from build123d import *

# Parameters (mm, degrees)
BOSS_EXTRUDE1_DEPTH     = 203.2
CUT_EXTRUDE3_DEPTH      = 17.51
CUT_EXTRUDE3_DEPTH_BACK = 4.175
SKETCH7_R               = 3.683
SKETCH7_R_2             = 1.63195
CUT_EXTRUDE4_DEPTH      = 20.685
SKETCH8_R               = 1.89865
CUT_EXTRUDE5_DEPTH      = 4.175
SKETCH9_R               = 1.89865
CUT_EXTRUDE6_DEPTH      = 4.175
SKETCH10_R              = 1.7526
CUT_EXTRUDE7_DEPTH      = 4.175
BOSS_EXTRUDE2_DEPTH     = 3.175
SKETCH12_R              = 2.54
CUT_EXTRUDE8_DEPTH      = 4.175
SKETCH13_R              = 1.89865
CUT_EXTRUDE9_DEPTH      = 4.175


with BuildPart() as part:
    # Sketch1 → Boss-Extrude1 (new body)
    with BuildSketch(Plane(origin=(0, 0, 0), x_dir=(1, 0, 0), z_dir=(0, 1, 0))):
        Polygon((0, 0), (-19.685, 0), (-19.685, 3.175), (-3.175, 3.175), (-3.175, 50.8), (0, 50.8), align=None)
    extrude(amount=BOSS_EXTRUDE1_DEPTH)

    # Sketch5 → Cut-Extrude3 (cut, two sides)
    with BuildSketch(Plane.ZY.offset(3.175)) as cut_extrude3_sk:
        Polygon((0, 163.322), (-50.8, 214.122), (-60.823247691, 214.122), (-60.823247691, 256.047203652), (33.196571846, 256.047203652), (33.196571846, 163.322), align=None)
    extrude(amount=CUT_EXTRUDE3_DEPTH, mode=Mode.SUBTRACT)
    extrude(cut_extrude3_sk.sketch, amount=-CUT_EXTRUDE3_DEPTH_BACK, mode=Mode.SUBTRACT)

    # Sketch7 → Cut-Extrude4 (cut, through all)
    with BuildSketch(Plane(origin=(0, 0, 0), x_dir=(0, 0, -1), z_dir=(1, 0, 0))):
        with Locations((25.4, 152.4)):
            Circle(SKETCH7_R)
        with Locations((25.4, 160.782)):
            Circle(SKETCH7_R_2)
        with Locations((25.4, 144.018)):
            Circle(SKETCH7_R_2)
    extrude(amount=-CUT_EXTRUDE4_DEPTH, mode=Mode.SUBTRACT)

    # Sketch8 → Cut-Extrude5 (cut, through all)
    with BuildSketch(Plane.ZY.offset(3.175)):
        with Locations((-30.48, 182.88)):
            Circle(SKETCH8_R)
        with Locations((-30.48, 8.89)):
            Circle(SKETCH8_R)
    extrude(amount=-CUT_EXTRUDE5_DEPTH, mode=Mode.SUBTRACT)

    # Sketch9 → Cut-Extrude6 (cut, through all)
    with BuildSketch(Plane.ZY.offset(3.175)):
        with Locations((-19.05, 40.577339992)):
            Circle(SKETCH9_R)
        with Locations((-19.05, 124.397339992)):
            Circle(SKETCH9_R)
    extrude(amount=-CUT_EXTRUDE6_DEPTH, mode=Mode.SUBTRACT)

    # Sketch10 → Cut-Extrude7 (cut, through all)
    with BuildSketch(Plane(origin=(0, 0, -3.175), x_dir=(-1, 0, 0), z_dir=(0, 0, -1))):
        with Locations((9.525, 11.43)):
            Circle(SKETCH10_R)
        with Locations((9.525, 150.603948776)):
            Circle(SKETCH10_R)
    extrude(amount=-CUT_EXTRUDE7_DEPTH, mode=Mode.SUBTRACT)

    # Sketch11 → Boss-Extrude2 (add)
    with BuildSketch(Plane(origin=(0, 0, 0), x_dir=(0, 0, -1), z_dir=(1, 0, 0))):
        Polygon((0, 228.6), (0, 163.322), (39.878, 203.2), (50.8, 203.2), (50.8, 228.6), align=None)
    extrude(amount=-BOSS_EXTRUDE2_DEPTH)

    # Sketch12 → Cut-Extrude8 (cut, through all)
    with BuildSketch(Plane.ZY.offset(3.175)):
        with Locations((-33.136196499, 25.4)):
            Circle(SKETCH12_R)
    extrude(amount=-CUT_EXTRUDE8_DEPTH, mode=Mode.SUBTRACT)

    # Sketch13 → Cut-Extrude9 (cut, through all)
    with BuildSketch(Plane.ZY.offset(3.175)):
        with Locations((-43.18, 12.7)):
            Circle(SKETCH13_R)
        with Locations((-43.18, 190.498941664)):
            Circle(SKETCH13_R)
    extrude(amount=-CUT_EXTRUDE9_DEPTH, mode=Mode.SUBTRACT)


solid = part.part
CAD build for the part. Positions are in the model's coordinates, mm. A direction names the side the tool comes from. Round coordinates to 2 decimals unless told otherwise and drop trailing zeros. Order: outer loops, then holes, each group sorted by start corner. A loop starts at its lowest first (then second) coordinate and runs counter-clockwise, first axis right, second up. Notation, with made-up numbers: (50, 7) -> (82, 7) arc R20 cw to (82, 38) -> close; hole circle Ø5 at (-26, 86). An arc over 180 degrees is marked (long way). Write item = value, one per line. Start each with the question number.
(1) Pin check, flat tips, straight feed: P1, Ø3, axis at y = 185.5, z = -19, coming from the +X side; P2, Ø4, axis at y = 144.018, z = -25.4, coming from the -X side (3 decimals); P3, Ø2, axis at x = -7.5, y = 82.5, coming from the -Z side (3 decimals); P4, Ø3, axis at x = -9.5, y = 165.5, coming from the +Z side. Stop position of each tip, or through.
(2) Cut at C-C, the plane y = 25.4. List the corners of the cut face in (x, z) (3 decimals), then the cut area to 3 significant figures.
(3) Pull direction Y, two halves, no side cores. Call faces 1 (the flat face through (0, 116, -25)), 2 (the cylindrical face through (-1.61, 126.28, -19.3)), 3 (the flat face through (-3, 0, -20)): released by +Y, released by -Y, zero draft, split by the parting line, or undercut.
(4) Which spindle directions (+Z, -Z, +X, -X, +Y, -Y) get a long thin tool onto all of the face, cutting with end or side? Do faces 4 (the flat face through (-12, 82, -3.175)), 5 (the cylindrical face through (-1.565, 149.133, -27.099)). Say none if no direction does.
(5) Cut at A-A, the plane z = -19.05. List the corners of the cut face in (x, y) (3 decimals).
(6) Probe line 1 (Y direction, x = -2.3, z = -30.48); line 2 (Y direction, x = -1.35, z = -19.05); line 3 (Y direction, x = -0.75, z = -25.4). List the from-to ranges inside material, lowest first. Write a range as [from, to].
(7) Cut at B-B, the plane y = 182.88. List the corners of the cut face in (x, z) (3 decimals).
(8) Cut at D-D, the plane x = -16. List the corners of the cut face in (y, z) (3 decimals).
Model answer:
q1.P1 = 0
q1.P2 = -3.175
q1.P3 = -3.175
q1.P4 = -0.68
q2.outline = (-19.685, -3.175) -> (-3.175, -3.175) -> (-3.175, -30.596) -> (0, -30.596) -> (0, 0) -> (-19.685, 0) -> close; (-3.175, -50.8) -> (0, -50.8) -> (0, -35.676) -> (-3.175, -35.676) -> close
q2.area = 198 mm2
q3.face_1 = zero draft
q3.face_2 = undercut
q3.face_3 = released by -Y
q4.face_4 = -Z, -X, +Y, -Y
q4.face_5 = +X, -X
q5.outline = (-3.175, 0) -> (0, 0) -> (0, 38.679) -> (-3.175, 38.679) -> close; (-3.175, 42.476) -> (0, 42.476) -> (0, 122.499) -> (-3.175, 122.499) -> close; (-3.175, 126.296) -> (0, 126.296) -> (0, 228.6) -> (-3.175, 228.6) -> close
q6.line_1 = [0, 6.99], [10.79, 180.98], [184.78, 228.6]
q6.line_2 = [0, 38.68], [42.48, 122.5], [126.3, 228.6]
q6.line_3 = [0, 142.39], [145.65, 148.72], [156.08, 159.15], [162.41, 228.6]
q7.outline = (-3.175, -50.8) -> (0, -50.8) -> (0, -32.379) -> (-3.175, -32.379) -> close; (-3.175, -28.581) -> (0, -28.581) -> (0, 0) -> (-3.175, 0) -> close
q8.outline = (0, -3.175) -> (166.497, -3.175) -> (163.322, 0) -> (0, 0) -> close
